from build123d import *

# Parameters (mm, degrees)
SKETCH1_W               = 203.2
SKETCH1_H               = 190.5
BOSS_EXTRUDE1_DEPTH     = 6.35
SKETCH2_W               = 12.7
SKETCH2_H               = 6.35
CUT_EXTRUDE1_DEPTH      = 7.35
LPATTERN1_COUNT         = 8
LPATTERN1_PITCH         = 25.4
MIRROR1_COPY_1_SKETCH_W = 12.7
MIRROR1_COPY_1_SKETCH_H = 6.35
MIRROR1_COPY_1_DEPTH    = 7.35
MIRROR1_COPY_2_SKETCH_W = 12.7
MIRROR1_COPY_2_SKETCH_H = 6.35
MIRROR1_COPY_2_DEPTH    = 7.35
MIRROR1_COPY_3_SKETCH_W = 12.7
MIRROR1_COPY_3_SKETCH_H = 6.35
MIRROR1_COPY_3_DEPTH    = 7.35
MIRROR1_COPY_4_SKETCH_W = 12.7
MIRROR1_COPY_4_SKETCH_H = 6.35
MIRROR1_COPY_4_DEPTH    = 7.35
MIRROR1_COPY_5_SKETCH_W = 12.7
MIRROR1_COPY_5_SKETCH_H = 6.35
MIRROR1_COPY_5_DEPTH    = 7.35
MIRROR1_COPY_6_SKETCH_W = 12.7
MIRROR1_COPY_6_SKETCH_H = 6.35
MIRROR1_COPY_6_DEPTH    = 7.35
MIRROR1_COPY_7_SKETCH_W = 12.7
MIRROR1_COPY_7_SKETCH_H = 6.35
MIRROR1_COPY_7_DEPTH    = 7.35
SKETCH4_W               = 6.35
SKETCH4_H               = 12.7
CUT_EXTRUDE2_DEPTH      = 7.35
LPATTERN2_COUNT         = 7
LPATTERN2_PITCH         = 25.4


with BuildPart() as part:
    # Sketch1 → Boss-Extrude1 (new body)
    with BuildSketch(Plane(origin=(0, 0, 0), x_dir=(1, 0, 0), z_dir=(0, 1, 0))):
        Rectangle(SKETCH1_W, SKETCH1_H)
    extrude(amount=BOSS_EXTRUDE1_DEPTH)

    # Sketch2 → Cut-Extrude1 (cut, through all)
    with BuildSketch(Plane.XZ):
        with Locations((-82.55, 92.075)):
            Rectangle(SKETCH2_W, SKETCH2_H)
    cut_extrude1 = extrude(amount=-CUT_EXTRUDE1_DEPTH, mode=Mode.SUBTRACT)

    # LPattern1: Cut-Extrude1 ×8
    with Locations(*[(i * LPATTERN1_PITCH, 0, 0) for i in range(1, LPATTERN1_COUNT)]):
        add(cut_extrude1, mode=Mode.SUBTRACT)

    # Mirror1: Cut-Extrude1 across plane
    add(cut_extrude1.mirror(Plane.XY), mode=Mode.SUBTRACT)

    # Mirror1 copy 1 sketch → Mirror1 copy 1 (cut, through all)
    with BuildSketch(Plane(origin=(25.4, 0, 0), x_dir=(1, 0, 0), z_dir=(0, -1, 0))):
        with Locations((-82.55, -92.075)):
            Rectangle(MIRROR1_COPY_1_SKETCH_W, MIRROR1_COPY_1_SKETCH_H)
    extrude(amount=-MIRROR1_COPY_1_DEPTH, mode=Mode.SUBTRACT)

    # Mirror1 copy 2 sketch → Mirror1 copy 2 (cut, through all)
    with BuildSketch(Plane(origin=(50.8, 0, 0), x_dir=(1, 0, 0), z_dir=(0, -1, 0))):
        with Locations((-82.55, -92.075)):
            Rectangle(MIRROR1_COPY_2_SKETCH_W, MIRROR1_COPY_2_SKETCH_H)
    extrude(amount=-MIRROR1_COPY_2_DEPTH, mode=Mode.SUBTRACT)

    # Mirror1 copy 3 sketch → Mirror1 copy 3 (cut, through all)
    with BuildSketch(Plane(origin=(76.2, 0, 0), x_dir=(1, 0, 0), z_dir=(0, -1, 0))):
        with Locations((-82.55, -92.075)):
            Rectangle(MIRROR1_COPY_3_SKETCH_W, MIRROR1_COPY_3_SKETCH_H)
    extrude(amount=-MIRROR1_COPY_3_DEPTH, mode=Mode.SUBTRACT)

    # Mirror1 copy 4 sketch → Mirror1 copy 4 (cut, through all)
    with BuildSketch(Plane(origin=(101.6, 0, 0), x_dir=(1, 0, 0), z_dir=(0, -1, 0))):
        with Locations((-82.55, -92.075)):
            Rectangle(MIRROR1_COPY_4_SKETCH_W, MIRROR1_COPY_4_SKETCH_H)
    extrude(amount=-MIRROR1_COPY_4_DEPTH, mode=Mode.SUBTRACT)

    # Mirror1 copy 5 sketch → Mirror1 copy 5 (cut, through all)
    with BuildSketch(Plane(origin=(127, 0, 0), x_dir=(1, 0, 0), z_dir=(0, -1, 0))):
        with Locations((-82.55, -92.075)):
            Rectangle(MIRROR1_COPY_5_SKETCH_W, MIRROR1_COPY_5_SKETCH_H)
    extrude(amount=-MIRROR1_COPY_5_DEPTH, mode=Mode.SUBTRACT)

    # Mirror1 copy 6 sketch → Mirror1 copy 6 (cut, through all)
    with BuildSketch(Plane(origin=(152.4, 0, 0), x_dir=(1, 0, 0), z_dir=(0, -1, 0))):
        with Locations((-82.55, -92.075)):
            Rectangle(MIRROR1_COPY_6_SKETCH_W, MIRROR1_COPY_6_SKETCH_H)
    extrude(amount=-MIRROR1_COPY_6_DEPTH, mode=Mode.SUBTRACT)

    # Mirror1 copy 7 sketch → Mirror1 copy 7 (cut, through all)
    with BuildSketch(Plane(origin=(177.8, 0, 0), x_dir=(1, 0, 0), z_dir=(0, -1, 0))):
        with Locations((-82.55, -92.075)):
            Rectangle(MIRROR1_COPY_7_SKETCH_W, MIRROR1_COPY_7_SKETCH_H)
    extrude(amount=-MIRROR1_COPY_7_DEPTH, mode=Mode.SUBTRACT)

    # Sketch4 → Cut-Extrude2 (cut, through all)
    with BuildSketch(Plane(origin=(0, 6.35, 0), x_dir=(1, 0, 0), z_dir=(0, 1, 0))):
        with Locations((98.425, 69.85)):
            Rectangle(SKETCH4_W, SKETCH4_H)
    cut_extrude2 = extrude(amount=-CUT_EXTRUDE2_DEPTH, mode=Mode.SUBTRACT)

    # LPattern2: Cut-Extrude2 ×7
    with Locations(*[(0, 0, i * LPATTERN2_PITCH) for i in range(1, LPATTERN2_COUNT)]):
        add(cut_extrude2, mode=Mode.SUBTRACT)


solid = part.part
Read the model definition and answer for the solid it produces. Units are mm, in the model's axes. A direction names the side the tool comes from. Give positions to 0.01 mm unless a question says otherwise; leave off trailing zeros. Write each loop counter-clockwise with the first axis right and the second up, starting at its lowest first coordinate (ties: lowest second). Pieces come first, ordered by that corner, then holes. Notation, with made-up numbers: (58, 80.25) - (81, 80.25) arc R14 cw to (81, 99.25) - close; hole circle Ø11 at (-27, 87). An arc over 180 degrees is marked (long way). Answer in a Markdown table with one row per item. Add a question column.
Item 1: A tool of negligible diameter and unlimited length cuts with its end or side. For faces 1 (the face through (88.9, 3, -92)), 2 (the face through (101.6, 3, 45)), 3 (the face through (6, 3, -95.25)), 4 (the face through (0, 3, -92)), 5 (the face through (95.25, 3, -19)), from which of +Z, -Z, +X, -X, +Y, -Y can it reach the whole face along a straight path? Write none if from no direction.
Item 2: Section B-B, the plane x = 23 is taken. Write down the section's boundary in (y, z).
Item 3: Determine the mould class of faces 6 (the face through (95.25, 3, -44)), 7 (the face through (-1, 6.35, -1)), 8 (the face through (-88.9, 3, 92)) for opening direction X: pulls with the +X half, pulls with the -X half, needs draft (parallel to the pull), parting line crosses it, or undercut.
Item 4: Section A-A, the plane z = -68 is taken. Write down the section's boundary in (x, y), and give its area (3 significant figures).
Item 5: Find the intervals of material crossed by L1, parallel to X at y = 1.5, z = -48; L2, parallel to Z at x = -86.5, y = 0.75, in increasing order.
Item 6: Flat-ended cylindrical pins translate along their axes: P1, Ø3, axis at y = 2.5, z = 90.5, coming from the +X side; P2, Ø3, axis at x = 98, y = 2.5, coming from the -Z side; P3, Ø1.9, axis at x = 42.5, y = 2.5, coming from the +Z side; P4, Ø10, axis at x = 19.5, z = -73, coming from the -Y side. Find the tip coordinate at first contact, or state that the pin passes through.
Recorded:
| question | item | result |
|---|---|---|
| 1 | face 1 | -Z, +X, +Y, -Y |
| 1 | face 2 | +Z, -Z, +X, +Y, -Y |
| 1 | face 3 | -Z, +X, -X, +Y, -Y |
| 1 | face 4 | -Z, +Y, -Y |
| 1 | face 5 | +X, +Y, -Y |
| 2 | outline | (0, -88.9) - (6.35, -88.9) - (6.35, 88.9) - (0, 88.9) - close |
| 3 | face 6 | pulls with the +X half |
| 3 | face 7 | needs draft |
| 3 | face 8 | undercut |
| 4 | outline | (-101.6, 0) - (95.25, 0) - (95.25, 6.35) - (-101.6, 6.35) - close |
| 4 | area | 1,250 mm2 |
| 5 | L1 | x = -101.6 to 95.25 |
| 5 | L2 | z = -88.9 to 88.9 |
| 6 | P1 | stops at x = 88.9 |
| 6 | P2 | stops at z = -88.9 |
| 6 | P3 | stops at z = 88.9 |
| 6 | P4 | stops at y = 0 |
